CAD build for the part. Positions are in the model's coordinates, mm. Face numbers are marked on the shaded views. A direction names the side the tool comes from. Give positions to 0.01 mm unless a question says otherwise; leave off trailing zeros. Write each loop counter-clockwise with the first axis right and the second up, starting at its lowest first coordinate (ties: lowest second). Pieces come first, ordered by that corner, then holes. Notation, with made-up numbers: (39.25, -0.75) - (89.25, -0.75) arc R20 cw to (89.25, 29.25) - close; hole circle Ø5 at (9, 67.25). An arc over 180 degrees is marked (long way). Answer as a JSON object with one key per item and string values.
from build123d import *

# Parameters (mm, degrees)
SKETCH1_W                    = 810
SKETCH1_H                    = 1020
BASE_FLANGE1_DEPTH           = 0.8
EDGE_FLANGE1_STRIP_W         = 4.8
EDGE_FLANGE1_STRIP_H         = 0.8
EDGE_FLANGE1_STRIP_CUT_DEPTH = 1020
EDGE_FLANGE1_DEPTH           = 1020
CUT_EXTRUDE2_DEPTH           = 10


# Sheet-metal steps are written as plain solids
with BuildPart() as part:
    # Sketch1 → Base-Flange1 (new body)
    with BuildSketch(Plane(origin=(0, 0, 0), x_dir=(1, 0, 0), z_dir=(0, 1, 0))):
        Rectangle(SKETCH1_W, SKETCH1_H)
    extrude(amount=-BASE_FLANGE1_DEPTH)

    # Edge-Flange1 strip (across the edge) → Edge-Flange1 strip cut (cut)
    with BuildSketch(Plane(origin=(-405, -0.8, 510), x_dir=(1, 0, 0), z_dir=(0, 0, -1))):
        with Locations((-0.8, -0.4)):
            Rectangle(EDGE_FLANGE1_STRIP_W, EDGE_FLANGE1_STRIP_H)
    extrude(amount=EDGE_FLANGE1_STRIP_CUT_DEPTH, mode=Mode.SUBTRACT)

    # Edge-Flange1 section (across the edge) → Edge-Flange1 (add)
    with BuildSketch(Plane(origin=(-405, -0.8, 510), x_dir=(1, 0, 0), z_dir=(0, 0, -1))):
        with BuildLine():
            Line((0, 0.8), (0, 40))
            Line((0, 40), (0.8, 40))
            Line((0.8, 40), (0.8, 0.8))
            ThreePointArc((0.8, 0.8), (1.034314575, 0.234314575), (1.6, 0))
            Line((1.6, 0), (1.6, -0.8))
            ThreePointArc((1.6, -0.8), (0.46862915, -0.33137085), (0, 0.8))
        make_face()
    extrude(amount=EDGE_FLANGE1_DEPTH)

    # Sketch7 → Cut-Extrude2 (cut)
    with BuildSketch(Plane(origin=(0, 0, 0), x_dir=(1, 0, 0), z_dir=(0, 1, 0))):
        with BuildLine():
            Line((405, 510), (367, 510))
            ThreePointArc((367, 510), (393.870057685, 498.870057685), (405, 472))
            Line((405, 472), (405, 510))
        make_face()
        with BuildLine():
            Line((405, -510), (367, -510))
            ThreePointArc((367, -510), (393.870057685, -498.870057685), (405, -472))
            Line((405, -472), (405, -510))
        make_face()
    extrude(amount=-CUT_EXTRUDE2_DEPTH, mode=Mode.SUBTRACT)


solid = part.part
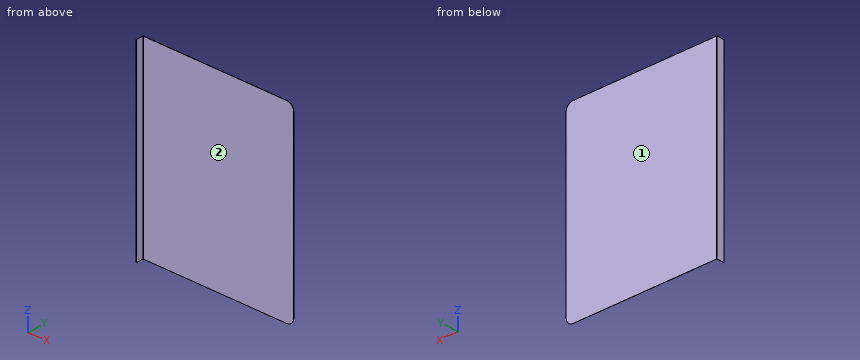
(1) Saw through at C-C, the plane x = -240. Give the cut face in (y, z).
Answer key:
{"outline": "(-0.8, -510) - (0, -510) - (0, 510) - (-0.8, 510) - close"}
(2) Saw through at B-B, the plane y = -34. Give the cut face in (x, z), and give its area (3 significant figures).
Answer key:
{"outline": "(-405, -510) - (-404.2, -510) - (-404.2, 510) - (-405, 510) - close", "area": "816 mm²"}
(3) Flat gauge pins, fed straight in: P1, Ø3, axis at x = 221.5, z = -326.5, coming from the -Y side; P2, Ø19.5, axis at y = -16.5, z = 100.5, coming from the +X side. Where does each tip first touch, or does it go through?
Answer key:
{"P1": "stops at y = -0.8", "P2": "stops at x = -404.2"}
(4) Saw through at A-A, the plane z = 410. Give the cut face in (x, y).
Answer key:
{"outline": "(-405, -40.8) - (-404.2, -40.8) - (-404.2, -1.6) arc R0.8 cw to (-403.4, -0.8) - (405, -0.8) - (405, 0) - (-403.4, 0) arc R1.6 ccw to (-405, -1.6) - close"}
(5) Probe L1, parallel to X at y = -5.5, z = 170.5; L2, parallel to Y at x = -153, z = -410. List the from-to ranges inside material, lowest first. Write a range as [from, to].
Answer key:
{"L1": "x = [-405, -404.2]", "L2": "y = [-0.8, 0]"}
(6) 3-axis set-ups, long thin cutter, end or side, ignore diameter. For the marked faces 1 and 2: which of +Z, -Z, +X, -X, +Y, -Y reach the whole face in a straight line?
Answer key:
{"face 1": "+Z, -Z, +X, -X, +Y", "face 2": "+Z, -Z, +X, -Y"}
